For this review, take the finished solid that the model builds, in its own axes (mm). A direction names the side the tool comes from. Give positions to 0.01 mm unless a question says otherwise; leave off trailing zeros. Loops run counter-clockwise (first coordinate to the right, second up) from the corner with the lowest first, then second, coordinate; pieces in that order, holes last.
```python
from build123d import *

# Parameters (mm, degrees)
F0_R           = 6.260280421
F1_DEPTH       = 10
F1_DEPTH_BACK  = 50
F1_FACE_R      = 6.260280421
F2_DEPTH       = 5
F2_TAPER       = 10
F1_FACE1_R     = 6.260280421
F3_DEPTH       = 5
F3_TAPER       = 10
F4_R           = 2.1661571195
F5_DEPTH       = 5
F5_TAPER       = -20
F6_R           = 3.8309083686
F7_DEPTH       = 5
F7_TAPER       = 20
F8_W           = 2.4537248537
F8_H           = 9.1121047735
F9_DEPTH       = 7
F9_DEPTH_BACK  = 7
F10_W          = 2.3227367783
F10_H          = 8.6134821177
F11_DEPTH      = 7
F11_DEPTH_BACK = 7


with BuildPart() as f1:
    # F0 (on Top) → F1 (new body, two sides)
    with BuildSketch(Plane.XY) as f1_sk:
        Circle(F0_R)
    extrude(amount=F1_DEPTH)
    extrude(f1_sk.sketch, amount=-F1_DEPTH_BACK)

    # F1_face (on face) → F2 (join)
    with BuildSketch(Plane.XY.offset(10)):
        Circle(F1_FACE_R)
    extrude(amount=F2_DEPTH, taper=F2_TAPER)

    # F1_face1 (on face) → F3 (join)
    with BuildSketch(Plane(origin=(0, 0, -50), x_dir=(1, 0, 0), z_dir=(0, 0, -1))):
        Circle(F1_FACE1_R)
    extrude(amount=F3_DEPTH, taper=F3_TAPER)

    # F4 (on face) → F5 (join)
    with BuildSketch(Plane(origin=(0, 0, -55), x_dir=(1, 0, 0), z_dir=(0, 0, -1))):
        Circle(F4_R)
    extrude(amount=F5_DEPTH, taper=F5_TAPER)

    # F6 (on face) → F7 (cut)
    with BuildSketch(Plane(origin=(0, 0, -60), x_dir=(1, 0, 0), z_dir=(0, 0, -1))):
        Circle(F6_R)
    extrude(amount=-F7_DEPTH, taper=F7_TAPER, mode=Mode.SUBTRACT)

    # F8 (on Front) → F9 (join, two sides)
    with BuildSketch(Plane.XZ) as f9_sk:
        with Locations((0.0925256172, -43.8020937145)):
            Rectangle(F8_W, F8_H)
    extrude(amount=F9_DEPTH)
    extrude(f9_sk.sketch, amount=-F9_DEPTH_BACK)

    # F10 (on Right) → F11 (join, two sides)
    with BuildSketch(Plane.YZ) as f11_sk:
        with Locations((-0.1453745062, -43.9728200436)):
            Rectangle(F10_W, F10_H)
    extrude(amount=F11_DEPTH)
    extrude(f11_sk.sketch, amount=-F11_DEPTH_BACK)


solid = f1.part
```
Item 1: Tool access review of faces 4 (the flat face through (2.3, 1.1, -55)), 5 (the conical face through (5.358, -1.687, -53.646)): name each direction out of +Z, -Z, +X, -X, +Y, -Y from which nothing blocks a thin tool from reaching the whole face with its end or side.
Answer:
face 4: none
face 5: -Z
Item 2: Take a section at B-B on z = 6. Give the boundary of the cut face in (x, y).
Answer:
outline: circle Ø12.52 at (0, 0)
Item 3: The part is to be moulded in two halves that separate along Y. For faces 1 (the flat face through (0, 0, -55)), 2 (the conical face through (-5.61, 0.25, 13.65)), 3 (the flat face through (0, -7, -44)), say which applies: released by +Y, released by -Y, zero draft, split by the parting line, or undercut.
Answer:
face 1: undercut
face 2: split by the parting line
face 3: released by -Y
Item 4: Clearance check with flat-ended pins moving along their axes: pin 1 Ø3 at (x, z) = (4.5, -1) entering from +Y; pin 2 Ø2 at (x, y) = (0.5, 0) entering from -Z; pin 3 Ø1.5 at (x, z) = (-4.5, -13) entering from +Y; pin 4 Ø4 at (x, z) = (-1.5, -48) entering from -Y. State where each tip first meets the part, or that it passes through.
Answer:
pin 1: stops at y = 5.49
pin 2: stops at z = -55
pin 3: stops at y = 5.01
pin 4: stops at y = -7
Item 5: Take a section at A-A on x = 0. Give the boundary of the cut face in (y, z).
Answer:
outline: (-7, -48.36) - (-6.26, -48.36) - (-6.26, -50) - (-5.38, -55) - (-2.17, -55) - (-3.99, -60) - (-3.83, -60) - (-2.01, -55) - (2.01, -55) - (3.83, -60) - (3.99, -60) - (2.17, -55) - (5.38, -55) - (6.26, -50) - (6.26, -48.36) - (7, -48.36) - (7, -39.25) - (6.26, -39.25) - (6.26, 10) - (5.38, 15) - (-5.38, 15) - (-6.26, 10) - (-6.26, -39.25) - (-7, -39.25) - close
Item 6: For L1, parallel to X at y = -1, z = 6; L2, parallel to Z at x = 1.75, y = 0.5; L3, parallel to Z at x = 1.75, y = 2.75, list the stretches that pass through material, from the lowest coordinate up.
Answer:
L1: x = -6.18 to 6.18
L2: z = -55 to 15
L3: z = -58.43 to -58, -55 to 15
